from build123d import *

# Parameters (mm, degrees)
F1_DEPTH = 1.016
F3_D     = 4.826


with BuildPart() as f1:
    # F0 (on Top) → F1 (new body)
    with BuildSketch(Plane.XY):
        with BuildLine():
            Line((-90.4505589354, 0), (-16.7905589354, 0))
            ThreePointArc((-16.7905589354, 0), (15.3250850137, 6.8603672412), (-11.1844753183, -12.5231937307))
            Line((-11.1844753183, -12.5231937307), (-60.2506472734, -67.4623088462))
            ThreePointArc((-60.2506472734, -67.4623088462), (82.5560668086, 36.9567239459), (-90.4505589354, 0))
        make_face()
        Polygon((-60.2506472734, -67.4623088462), (-11.1844753183, -12.5231937307), (-20.6567365451, -4.0635089109), (-69.7229085002, -59.0026240263), align=None)
    extrude(amount=F1_DEPTH)

    # F3 (through all)
    with Locations(Plane(origin=(0, 0, 0), x_dir=(1, 0, 0), z_dir=(0, 0, -1))):
        with Locations((-77.7505589354, -6.35), (-52.3505589354, -6.35), (-26.9505589354, -6.35), (-22.6883537876, 15.8711603022), (-39.6077234273, 34.8156827558), (-56.5270930669, 53.7602052095)):
            Hole(F3_D / 2)


solid = f1.part
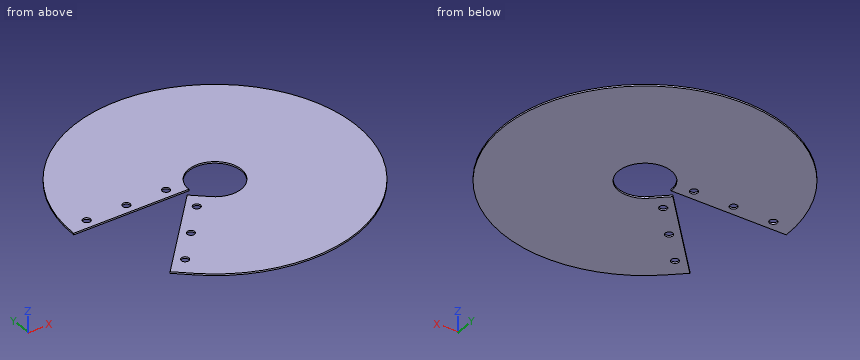
Read the model definition and answer for the solid it produces. Units are mm, in the model's axes. Give positions to 0.01 mm unless a question says otherwise; leave off trailing zeros. Loops run counter-clockwise (first coordinate to the right, second up) from the corner with the lowest first, then second, coordinate; pieces in that order, holes last. Notation, with made-up numbers: M 19.25,-18.75 L 34.25,-18.75 A26 ccw 34.25,13.25 Z; hole C 11,-8.75 d7. An arc over 180 degrees is marked long. Write each question's results on one line, items separated by ' | '.
1. Section D-D on y = -29 is taken. Give the vertices of the cut face in (x, z), plus the area to 3 significant figures.
Values:
outline: M -42.93,0 L 85.68,0 L 85.68,1.02 L -42.93,1.02 Z | area: 131 mm^2
2. Section B-B on y = -7 is taken. Give the vertices of the cut face in (x, z).
Values:
outline: M -23.28,0 L -17.37,0 L -17.37,1.02 L -23.28,1.02 Z; M 15.26,0 L 90.18,0 L 90.18,1.02 L 15.26,1.02 Z
3. Section C-C on z = 0.7 is taken. Give the vertices of the cut face in (x, y), plus the area to 3 significant figures.
Values:
outline: M -90.45,0 L -16.79,0 A16.79 cw long -11.18,-12.52 L -20.66,-4.06 L -69.72,-59 L -60.25,-67.46 A90.45 ccw long Z; hole C -77.75,6.35 d4.83; hole C -56.53,-53.76 d4.83; hole C -52.35,6.35 d4.83; hole C -39.61,-34.82 d4.83; hole C -26.95,6.35 d4.83; hole C -22.69,-15.87 d4.83 | area: 22,300 mm^2
4. Section A-A on x = 0 is taken. Give the vertices of the cut face in (y, z), plus the area to 3 significant figures.
Values:
outline: M -90.45,0 L -16.79,0 L -16.79,1.02 L -90.45,1.02 Z; M 16.79,0 L 90.45,0 L 90.45,1.02 L 16.79,1.02 Z | area: 150 mm^2
5. Given pin 1 (0.5 mm diameter, centred on x = -37, z = 0.5, fed in from -Y), flat-ended and moving along its own axis, determine where the tip first touches the part or whether it passes through.
Values:
pin 1: stops at y = -82.65
6. Straight lines are drawn through the part: line 1 (Y direction, x = -4, z = 0.6); line 2 (Y direction, x = 11, z = 0.1); line 3 (X direction, y = 10, z = 0.3). For each, find the intervals that lie inside material, in ascending order. Write a range as [from, to].
Values:
line 1: y = [-90.36, -16.31], [16.31, 90.36] | line 2: y = [-89.78, -12.69], [12.69, 89.78] | line 3: x = [-89.9, -13.49], [13.49, 89.9]
